The listing builds one solid part. Answer for the finished solid, in the listing's coordinates (mm). A direction names the side the tool comes from. Coordinates: 2 decimals unless noted, no trailing zeros. Return JSON: item names as keys, results as strings.
from build123d import *

# Parameters (mm, degrees)
SKETCH5_R          = 200
CUT_EXTRUDE3_DEPTH = 201


with BuildPart() as part:
    # Sketch2 → Revolve2 (revolve)
    with BuildSketch(Plane.XY):
        with BuildLine():
            Line((60, 450), (60, 440))
            Line((60, 440), (80, 440))
            Line((80, 440), (80, 450))
            Line((80, 450), (100, 450))
            Line((100, 450), (100, 440))
            Line((100, 440), (120, 440))
            Line((120, 440), (120, 450))
            Line((120, 450), (140, 450))
            Line((140, 450), (140, 440))
            Line((140, 440), (160, 440))
            Line((160, 440), (160, 450))
            Line((160, 450), (180, 450))
            Line((180, 450), (180, 440))
            Line((180, 440), (200, 440))
            Line((200, 440), (200, 450))
            Line((200, 450), (220, 450))
            Line((220, 450), (220, 440))
            Line((220, 440), (240, 440))
            Line((240, 440), (240, 450))
            Line((240, 450), (250, 450))
            ThreePointArc((250, 450), (285.355339059, 435.355339059), (300, 400))
            Line((300, 400), (300, 341.421356237))
            ThreePointArc((300, 341.421356237), (272.474487139, 254.818815859), (200, 200))
            Line((200, 200), (200, 0))
            Line((200, 0), (100, 0))
            Line((100, 0), (100, 200))
            ThreePointArc((100, 200), (27.525512861, 254.818815859), (0, 341.421356237))
            Line((0, 341.421356237), (0, 400))
            ThreePointArc((0, 400), (14.644660941, 435.355339059), (50, 450))
            Line((50, 450), (60, 450))
        make_face()
    revolve(axis=Axis((100, 0, 0), (1, 0, 0)))

    # Sketch5 → Cut-Extrude3 (cut, through all)
    with BuildSketch(Plane.ZY.offset(-100)):
        Circle(SKETCH5_R)
    extrude(amount=-CUT_EXTRUDE3_DEPTH, mode=Mode.SUBTRACT)


solid = part.part
1. Determine the mould class of faces 3 (the face through (0, -294, 180)), 4 (the face through (300, 294, 180)), 5 (the face through (80, -431, -98)), 6 (the face through (149.3, 60.075, 190.764)) for opening direction X: pulls with the +X half, pulls with the -X half, needs draft (parallel to the pull), parting line crosses it, or undercut.
Answer block:
{"face 3": "pulls with the -X half", "face 4": "pulls with the +X half", "face 5": "undercut", "face 6": "needs draft"}
2. Each of these flat-tipped pins is pushed along its axis until it touches: pin 1 Ø1.5 at (y, z) = (-255.5, -45.5) entering from +X; pin 2 Ø1.5 at (x, y) = (87.5, 171) entering from -Z; pin 3 Ø10 at (x, z) = (232, 103) entering from -Y. Where does it stop, or does it pass through?
Answer block:
{"pin 1": "stops at x = 276.15", "pin 2": "stops at z = -416.55", "pin 3": "stops at y = -428.95"}
3. Consider line 1 (Z direction, x = 158.5, y = 0); line 2 (Z direction, x = 175.5, y = 0); line 3 (Y direction, x = 258.5, z = 104). Determine where each line is inside the solid, lowest interval first. Write a range as from..to.
Answer block:
{"line 1": "z = -440..-200, 200..440", "line 2": "z = -450..-200, 200..450", "line 3": "y = -437.07..-213.9, 213.9..437.07"}
4. For faces 1 (the face through (140, 431, -98)), 2 (the face through (90.14, -449.565, 19.786)), determine the directions among +Z, -Z, +X, -X, +Y, -Y from which every point of the face is accessible in a straight line to the end or side of a thin tool.
Answer block:
{"face 1": "none", "face 2": "+X, -X"}
